Autodesk Inventor part; units mm, degrees
ref_plane "YZ Plane" through (0, 0, 0) normal (1, 0, 0) x (0, 1, 0)
ref_plane "XZ Plane" through (0, 0, 0) normal (0, 1, 0) x (-1, 0, 0)
ref_plane "XY Plane" through (0, 0, 0) normal (0, 0, 1) x (1, 0, 0)
sketch "Sketch4" plane through (0, 0, 0) normal (0, 1, 0) x (-1, 0, 0)
  line L0 (-13.6, -3.4347) -> (-13.6, -11.4347)
  line L1 (-11, -9.4347) -> (-10, -9.4347)
  line L2 (-11, -3.4347) -> (-10, -3.4347)
  line L3 (-10, -3.4347) -> (-10, -9.4347)
  line L4 (0, 0) -> (0, -21.3586) construction
  line L5 (-10, -11.4347) -> (-13.6, -11.4347)
  line L6 (-10, -1.4347) -> (-12, -1.4347)
  line L7 (-11, -9.4347) -> (-11, -10.4347)
  line L8 (-11, -10.4347) -> (-10, -10.4347)
  line L9 (-11, -3.4347) -> (-11, -2.4347)
  line L10 (-11, -2.4347) -> (-10, -2.4347)
  line L11 (-10, -1.4347) -> (-10, -2.4347)
  line L12 (-10, -10.4347) -> (-10, -11.4347)
  line L13 (-13.2, -1.4347) -> (-12, -1.4347)
  line L14 (-13.2, -3.0347) -> (-13.2, -1.4347)
  line L15 (-13.6, -3.4347) -> (-13, -3.4347)
  line L16 (-13, -3.4347) -> (-13, -3.0347)
  line L17 (-13, -3.0347) -> (-13.2, -3.0347)
  point P0 (-10, -10.9347)
  point P1 (-11, -9.9347)
  dimension "d23" = 8
  dimension "d28" = 6
  dimension "d29" = 10
  dimension "d37" = 1
  dimension "d38" = 1
  dimension "d39" = 10
  dimension "d40" = 11
  dimension "d41" = 11
  dimension "d42" = 1
  dimension "d43" = 10
  dimension "d44" = 2
  dimension "d63" = 0.6
  dimension "d64" = 13.6
  dimension "d65" = 13.2
revolve "Revolution1" add sketch "Sketch4" angle 360 about axis through (0, 0, 0) along (0, 0, -1)
chamfer "Chamfer1" distance 0.5 angle 45 1 edges at (-13.2, 0, -1.4347)
sketch "Sketch5" plane through (0, 0, -3.4347) normal (0, 0, 1) x (1, 0, 0)
  circle A0 centre (0, 0) radius 13.6
  point P0 (13.6, 0)
  point P1 (-13.6, 0)
ref_plane "Work Plane1" through (13.6, 0, -3.4347) normal (1, 0, 0) x (0, 1, 0)
ref_plane "Work Plane2" through (-13.6, 0, -3.4347) normal (-1, 0, 0) x (0, -1, 0)
chamfer "Chamfer2" distance 0.5 angle 45 1 edges at (-13.6, 0, -11.4347)
chamfer "Chamfer3" distance 0.2 angle 45 1 edges at (-10, 0, -1.4347)
chamfer "Chamfer4" distance 0.2 angle 45 1 edges at (-10, 0, -11.4347)
properties part number "tuleja łożyska"
Design review of the part built by this model. Coordinates are the model's own, in mm. A direction names the side the tool comes from. Round coordinates to 2 decimals unless told otherwise and drop trailing zeros. Write each loop counter-clockwise with the first axis right and the second up, starting at its lowest first coordinate (ties: lowest second). Pieces come first, ordered by that corner, then holes.
Item 1: Clearance check with flat-ended pins moving along their axes: pin 1 Ø8 at (x, y) = (0.5, -4) entering from -Z; pin 2 Ø6.5 at (x, y) = (5.5, -4) entering from +Z; pin 3 Ø1 at (y, z) = (-2.5, -9) entering from -X; pin 4 Ø2 at (y, z) = (-6, -5.5) entering from +X. State where each tip first meets the part, or that it passes through.
Item 2: The part is to be moulded in two halves that separate along Z. For faces 1 (the cylindrical face through (-2.17, 9.76, -10.84)), 2 (the cylindrical face through (-10.316, -7.91, -3.232)), 3 (the flat face through (-0.1, -10.4, -1.435)), say which applies: +Z half, -Z half, draft (parallel to the pull), parting line (faces both ways), or undercut.
Item 3: For probe 1 along Y at (x, z) = (0, -5.8); probe 2 along Z at (x, y) = (3.5, 9.75); probe 3 along X at (y, z) = (0, -9.85), list the stretches that pass through material, from the lowest coordinate up.
Item 4: We need section A-A on z = -7.25. Write out the cut boundary in (x, y), and give its area (3 significant figures).
Item 5: For faces 4 (the flat face through (2, 10, -3.435)), 5 (the cylindrical face through (-2.948, 13.277, -7.237)), 6 (the cylindrical face through (-9.73, 8.92, -2.48)), list the 3-axis set-ups (+Z, -Z, +X, -X, +Y, -Y) from which the entire face can be reached by the end or side of a thin tool; tool diameter is ignored.
Returned:
1. pin 1: passes through
1. pin 2: stops at z = -1.58
1. pin 3: stops at x = -13.45
1. pin 4: stops at x = 12.65
2. face 1: draft
2. face 2: undercut
2. face 3: +Z half
3. probe 1: y = -13.6 to -10, 10 to 13.6
3. probe 2: z = -11.43 to -10.43, -9.43 to -3.43, -2.43 to -1.43
3. probe 3: x = -13.6 to -11, 11 to 13.6
4. outline: circle Ø27.2 at (0, 0); hole circle Ø20 at (0, 0)
4. area: 267 mm2
5. face 4: none
5. face 5: +Z, -Z
5. face 6: +Z
